Geometry check sheet. Reference: the model listing, model coordinates, mm. Give positions to 0.01 mm unless a question says otherwise; leave off trailing zeros. Order: outer loops, then holes, each group sorted by start corner. A loop starts at its lowest first (then second) coordinate and runs counter-clockwise, first axis right, second up. Notation, with made-up numbers: M 33,24.5 L 86,24.5 A32 ccw 86,55.5 Z; hole C -12,-16.5 d7. An arc over 180 degrees is marked long. Answer as CSV lines item,"result".
from build123d import *

# Parameters (mm, degrees)
F1_DEPTH       = 10
F3_DEPTH       = 4
F5_D           = 4
F5_CSINK_D     = 7
F5_CSINK_ANGLE = 90
F6_R           = 3


with BuildPart() as f1:
    # F0 (on Front) → F1 (new body)
    with BuildSketch(Plane.XZ):
        Polygon((228.6, 24.4), (-24.4, 24.4), (0, 0), (204.2, 0), align=None)
    extrude(amount=F1_DEPTH)

    # F2 (on face) → F3 (cut)
    with BuildSketch(Plane.XZ.offset(10)):
        Polygon((-24.4, 9.5), (-24.4, 0), (0, 0), (-9.5, 9.5), align=None)
        Polygon((-9.5, 9.5), (0, 0), (204.2, 0), (213.7, 9.5), align=None)
        Polygon((213.7, 9.5), (204.2, 0), (228.6, 0), (228.6, 9.5), align=None)
    extrude(amount=-F3_DEPTH, mode=Mode.SUBTRACT)

    # F5 (through all)
    with Locations(Plane(origin=(0, 0, 0), x_dir=(-1, 0, 0), z_dir=(0, 1, 0))):
        with Locations((-188.6, 16), (-15.6, 16)):
            CounterSinkHole(F5_D / 2, F5_CSINK_D / 2, counter_sink_angle=F5_CSINK_ANGLE)

    # F6
    f6_edges = [f1.edges().sort_by_distance(p)[0] for p in [
        (102.1, 0, 0),
        (102.1, 0, 24.4),
    ]]
    fillet(f6_edges, radius=F6_R)


solid = f1.part
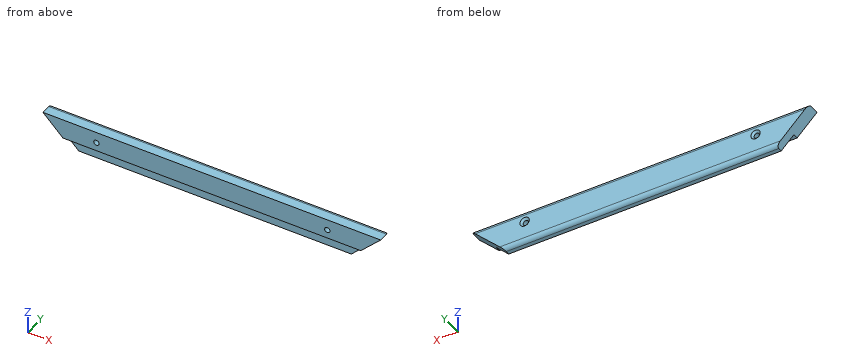
(1) Section check A-A on x = 141. Enter the section's corners in (y, z).
The answers:
outline,"M -10,9.5 L -6,9.5 L -6,0 L -3,0 A3 ccw 0,3 L 0,21.4 A3 ccw -3,24.4 L -10,24.4 Z"
(2) Section check B-B on z = 6. Enter the section's corners in (x, y), then the cut area to 3 significant figures.
The answers:
outline,"M -6,-6 L 210.2,-6 L 210.2,0 L -6,0 Z"
area,"1,300 mm2"
(3) Gauge pin test, flat ends, axial feed: P1, Ø4, axis at y = -6.5, z = 18, coming from the +X side; P2, Ø2, axis at x = 194, z = 6, coming from the -Y side; P3, Ø2, axis at y = -6, z = 13.5, coming from the -X side. Record the tip position at first contact, or that the pin passes through.
The answers:
P1,"stops at x = 224.2"
P2,"stops at y = -6"
P3,"stops at x = -14.5"
(4) Material ranges on line 1 (Z direction, x = 15.6, y = -5); line 2 (X direction, y = -5, z = 16); line 3 (Z direction, x = 188.6, y = -7.5), recorded low to high.
The answers:
line 1,"z = 0 to 14, 18 to 24.4"
line 2,"x = -16 to 13.6, 17.6 to 186.6, 190.6 to 220.2"
line 3,"z = 9.5 to 14, 18 to 24.4"
